The model under review builds one solid part; all positions refer to its coordinate system, in mm. Face numbers are marked on the shaded views. Give positions to 0.01 mm unless a question says otherwise; leave off trailing zeros. Loops run counter-clockwise (first coordinate to the right, second up) from the corner with the lowest first, then second, coordinate; pieces in that order, holes last. Notation, with made-up numbers: M 86.5,11.25 L 106.5,11.25 A16 cw 106.5,15.25 Z; hole C 18,14.5 d9. An arc over 180 degrees is marked long. Put each result on its own line as item: value. Start each with the question number.
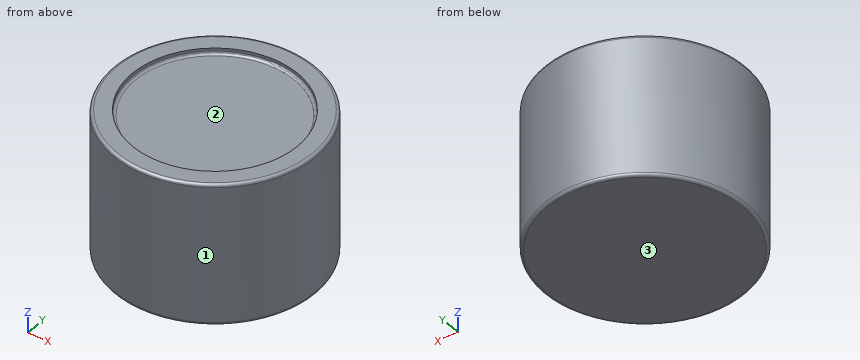
```python
from build123d import *

# Parameters (mm, degrees)
SKETCH_R        = 3.55
PAD_DEPTH       = 5
SKETCH004_R     = 2.912147
POCKET001_DEPTH = 0.2
FILLET001_R     = 0.1
FILLET002_R     = 0.1


with BuildPart() as part:
    # Sketch → Pad (new body)
    with BuildSketch(Plane.XY.offset(0.1)):
        Circle(SKETCH_R)
    extrude(amount=PAD_DEPTH)

    # Sketch004 → Pocket001 (cut)
    with BuildSketch(Plane.XY.offset(5.1)):
        Circle(SKETCH004_R)
    extrude(amount=-POCKET001_DEPTH, mode=Mode.SUBTRACT)

    # Fillet001
    fillet001_edges = [part.edges().sort_by_distance(p)[0] for p in [
        (-2.912147, 0, 4.9),
    ]]
    fillet(fillet001_edges, radius=FILLET001_R)

    # Fillet002
    fillet002_edges = [part.edges().sort_by_distance(p)[0] for p in [
        (-3.55, 0, 0.1),
        (-3.55, 0, 5.1),
    ]]
    fillet(fillet002_edges, radius=FILLET002_R)


solid = part.part
```
Item 1: Consider section C-C, the plane z = 3.9. Write out the cut boundary in (x, y).
Item 2: Draft analysis for pull direction X (two halves, no side actions). For the marked faces 1, 2 and 3, state which applies: +X half, -X half, draft (parallel to the pull), parting line (faces both ways), or undercut.
Item 3: Consider section A-A, the plane x = 0. Write out the cut boundary in (y, z), plus the area to 3 significant figures.
Item 4: To check wall thickness, follow L1, parallel to Z at x = 2.5, y = -0.5; L2, parallel to Z at x = -1.75, y = 3; L3, parallel to Y at x = 0.25, z = 2.6. State the ranges of each line that lie inside material, in increasing order. Write a range as [from, to].
Item 5: Clearance check with a flat-ended pin moving along its axis: pin 1 Ø1.7 at (x, y) = (-0.5, 1) entering from +Z. State where the tip first meets the part, or that it passes through.
Report:
1. outline: C 0,0 d7.1
2. face 1: parting line
2. face 2: undercut
2. face 3: draft
3. outline: M -3.55,0.2 A0.1 ccw -3.45,0.1 L 3.45,0.1 A0.1 ccw 3.55,0.2 L 3.55,5 A0.1 ccw 3.45,5.1 L 2.91,5.1 L 2.91,5 A0.1 cw 2.81,4.9 L -2.81,4.9 A0.1 cw -2.91,5 L -2.91,5.1 L -3.45,5.1 A0.1 ccw -3.55,5 Z
3. area: 34.3 mm²
4. L1: [0.1, 4.9]
4. L2: [0.1, 5.1]
4. L3: [-3.54, 3.54]
5. pin 1: z = 4.9
